The listing builds one solid part. Answer for the finished solid, in the listing's coordinates (mm). A direction names the side the tool comes from. Round coordinates to 2 decimals unless told otherwise and drop trailing zeros. Loops run counter-clockwise (first coordinate to the right, second up) from the corner with the lowest first, then second, coordinate; pieces in that order, holes last. Notation, with made-up numbers: (73.5, 60.25) -> (77.5, 60.25) arc R31 ccw to (77.5, 91.25) -> close; hole circle Ø1 at (57.5, 53.5). An arc over 180 degrees is marked (long way). Use a Markdown table: item, result. Add a question column.
Q1. Which of the six approach directions +Z, -Z, +X, -X, +Y, -Y give full straight-line access (tool end or side, diameter ignored) to faces 1 (the cylindrical face through (3.85, 12.62, 0.05)), 2 (the cylindrical face through (0, 5.1, -4.1)), 3 (the flat face through (1.1, 11.8, 1.4)), 4 (the cylindrical face through (0, 12.2, -4.1))?
Q2. Section B-B on z = 0 is taken. Give the vertices of the cut face in (x, y).
Q3. For a pull along X with two mould halves and no side action, classify faces 5 (the conical face through (3.56, 15.29, 0.05)), 6 (the cylindrical face through (0, 12.2, 4.1)), 7 (the cylindrical face through (2.462, 5.817, -1.69)) as released by +X, released by -X, zero draft, split by the parting line, or undercut.
Q4. Consider line 1 (X direction, y = 13.95, z = 0); line 2 (Y direction, x = 2, z = 1); line 3 (Z direction, x = 0, y = 5). Determine where each line is inside the solid, lowest interval first.
Q5. Section A-A on y = 12.25 is taken. Give the vertices of the cut face in (x, z) (3 decimals).
Q6. Section C-C on y = 2 is taken. Give the vertices of the cut face in (x, z) (3 decimals), then the cut area to 3 significant figures.
Q7. Given pin 1 Ø3 at (x, y) = (4, 7) entering from -Z; pin 2 Ø5 at (y, z) = (5, 2.5) entering from -X; pin 3 Ø1.5 at (x, y) = (1.5, 4.5) entering from -Z; pin 4 Ø1.4 at (x, z) = (-0.5, -0.5) entering from -Y (3 decimals), each flat-ended and moving along its own axis, determine where each tip first touches the part or whether it passes through.
from build123d import *

# Parameters (mm, degrees)
BOSS_EXTRUDE1_DEPTH = 15.4
CUT_EXTRUDE1_DEPTH  = 11.8
CUT_EXTRUDE2_REACH  = 18.939
SKETCH5_R           = 1.5
CHAMFER1_SIZE       = 0.4


with BuildPart() as part:
    # Sketch1 → Boss-Extrude1 (new body)
    with BuildSketch(Plane(origin=(0, 0, 0), x_dir=(1, 0, 0), z_dir=(0, 1, 0))):
        with BuildLine():
            ThreePointArc((-2.525, -3.23022832), (0, -4.1), (2.525, -3.23022832))
            ThreePointArc((2.525, -3.23022832), (3.85, 0), (2.525, 3.23022832))
            ThreePointArc((2.525, 3.23022832), (0, 4.1), (-2.525, 3.23022832))
            ThreePointArc((-2.525, 3.23022832), (-3.85, 0), (-2.525, -3.23022832))
        make_face()
    extrude(amount=BOSS_EXTRUDE1_DEPTH)

    # Sketch2 → Revolve1 (revolve)
    with BuildSketch(Plane.XY, mode=Mode.PRIVATE) as revolve1_sk:
        Polygon((3.85, 0), (3.85, 3.9), (2.35, 5.4), (-0.75, 5.4), (-0.75, 0), align=None)
    revolve(revolve1_sk.sketch.rotate(Axis((-0.75, 5.4, 0), (0, -1, 0)), 270), axis=Axis((-0.75, 5.4, 0), (0, -1, 0)))

    # Sketch3 → Revolve2 (revolve)
    with BuildSketch(Plane.XY, mode=Mode.PRIVATE) as revolve2_sk:
        Polygon((0.75, 4.8), (-2.35, 4.8), (-3.85, 6.3), (-3.85, 9.4), (-2.35, 10.9), (0.75, 10.9), align=None)
    revolve(revolve2_sk.sketch.rotate(Axis((0.75, 4.8, 0), (0, 1, 0)), 315.394327097), axis=Axis((0.75, 4.8, 0), (0, 1, 0)))

    # Sketch4 → Cut-Extrude1 (cut)
    with BuildSketch(Plane.XZ):
        with BuildLine():
            Line((-2, -2), (2, -2))
            ThreePointArc((2, -2), (2.465465068, -1.682598659), (2.339973189, -1.133369081))
            ThreePointArc((2.339973189, -1.133369081), (0, 2.6), (-2.339973189, -1.133369081))
            ThreePointArc((-2.339973189, -1.133369081), (-2.465465068, -1.682598659), (-2, -2))
        make_face()
    extrude(amount=-CUT_EXTRUDE1_DEPTH, mode=Mode.SUBTRACT)

    # Sketch5 → Cut-Extrude2 (cut, up to next)
    with BuildSketch(Plane(origin=(0, 15.4, 0), x_dir=(1, 0, 0), z_dir=(0, 1, 0)), mode=Mode.PRIVATE) as cut_extrude2_sk1:
        with Locations(Location((0, 0, 0), (0, 0, 270))):
            Circle(SKETCH5_R)
    cut_extrude2_tool1 = extrude(cut_extrude2_sk1.sketch, amount=-CUT_EXTRUDE2_REACH, mode=Mode.PRIVATE) & part.part
    add(cut_extrude2_tool1.solids().sort_by_distance((0, 15.4, 0))[0], mode=Mode.SUBTRACT)

    # Chamfer1
    # the kernel refuses this chamfer: 0.4 mm, written as the material it takes off along each edge
    with BuildSketch(Plane(origin=(0, 15.4, 0), x_dir=(-0.7922190522423981, 0, 0.6102368173620439), z_dir=(-0.6102368173620439, 0, -0.7922190522423981))) as chamfer1_piece_1:
        Polygon((4.1 - CHAMFER1_SIZE, 0), (4.1, -CHAMFER1_SIZE), (4.1, 0), align=None)
    revolve(axis=Axis((0, 15.4, 0), (0, 1, 0)), revolution_arc=104.786743256, mode=Mode.SUBTRACT)
    with BuildSketch(Plane(origin=(-0.75, 15.4, 0), x_dir=(0.5384255548923128, 0, 0.8426730812354843), z_dir=(-0.8426730812354843, 0, 0.5384255548923128))) as chamfer1_piece_2:
        Polygon((4.6 - CHAMFER1_SIZE, 0), (4.6, -CHAMFER1_SIZE), (4.6, 0), align=None)
    revolve(axis=Axis((-0.75, 15.4, 0), (0, 1, 0)), revolution_arc=114.846952535, mode=Mode.SUBTRACT)
    with BuildSketch(Plane(origin=(0, 15.4, 0), x_dir=(0.7922190522423987, 0, -0.610236817362043), z_dir=(0.610236817362043, 0, 0.7922190522423987))) as chamfer1_piece_3:
        Polygon((4.1 - CHAMFER1_SIZE, 0), (4.1, -CHAMFER1_SIZE), (4.1, 0), align=None)
    revolve(axis=Axis((0, 15.4, 0), (0, 1, 0)), revolution_arc=104.786743256, mode=Mode.SUBTRACT)
    with BuildSketch(Plane(origin=(0.75, 15.4, 0), x_dir=(-0.5384255548923127, 0, -0.8426730812354845), z_dir=(0.8426730812354845, 0, -0.5384255548923127))) as chamfer1_piece_4:
        Polygon((4.6 - CHAMFER1_SIZE, 0), (4.6, -CHAMFER1_SIZE), (4.6, 0), align=None)
    revolve(axis=Axis((0.75, 15.4, 0), (0, 1, 0)), revolution_arc=114.846952535, mode=Mode.SUBTRACT)


solid = part.part
Checked values:
| question | item | result |
|---|---|---|
| 1 | face 1 | +X, +Y |
| 1 | face 2 | -Z |
| 1 | face 3 | -Y |
| 1 | face 4 | -Z, +Y |
| 2 | outline | (-5.35, 0) -> (-2.6, 0) -> (-2.6, 11.8) -> (-1.5, 11.8) -> (-1.5, 15.4) -> (-3.45, 15.4) -> (-3.85, 15) -> (-3.85, 5.4) -> (-5.35, 3.9) -> close; (1.5, 11.8) -> (2.6, 11.8) -> (2.6, 0) -> (3.85, 0) -> (3.85, 4.8) -> (5.35, 6.3) -> (5.35, 9.4) -> (3.85, 10.9) -> (3.85, 15) -> (3.45, 15.4) -> (1.5, 15.4) -> close |
| 3 | face 5 | released by +X |
| 3 | face 6 | split by the parting line |
| 3 | face 7 | undercut |
| 4 | line 1 | x = -3.85 to -1.5, 1.5 to 3.85 |
| 4 | line 2 | y = 11.8 to 15.4 |
| 4 | line 3 | z = -4.1 to -2, 2.6 to 4.1 |
| 5 | outline | (-2.525, -3.23) arc R4.1 ccw to (2.525, -3.23) arc R4.6 ccw to (2.525, 3.23) arc R4.1 ccw to (-2.525, 3.23) arc R4.6 ccw to start; hole circle Ø3 at (0, 0) |
| 6 | outline | circle Ø9.2 at (-0.75, 0); hole (-2.34, -1.133) arc R0.5 ccw to (-2, -2) -> (2, -2) arc R0.5 ccw to (2.34, -1.133) arc R2.6 ccw (long way) to start |
| 6 | area | 46.0 mm2 |
| 7 | pin 1 | stops at z = -4.25 |
| 7 | pin 2 | stops at x = -5.34 |
| 7 | pin 3 | stops at z = -4.23 |
| 7 | pin 4 | passes through |
